from build123d import *

# Parameters (mm, degrees)
SALIENTE_EXTRUIR1_DEPTH = 5
CROQUIS3_W              = 12.5
CROQUIS3_H              = 5
SALIENTE_EXTRUIR2_DEPTH = 25
CROQUIS4_R              = 2.1
CORTAR_EXTRUIR3_DEPTH   = 12.5
CORTAR_EXTRUIR2_DEPTH   = 5.875


with BuildPart() as part:
    # Croquis2 → Saliente-Extruir1 (new body)
    with BuildSketch(Plane(origin=(0, 0, 0), x_dir=(1, 0, 0), z_dir=(0, 1, 0))):
        with BuildLine():
            Line((0, 0), (0, 12.5))
            Line((0, 12.5), (90, 35.865427318))
            add(Edge.make_bspline(
                [(0, 0), (0.394136999, 0.015797336), (1.194952966, 0.048834045), (2.992448828, 0.125211317), (4.579856068, 0.200911656), (6.612637351, 0.301249971), (8.392251736, 0.398752477), (10.315878033, 0.509903005), (12.159048858, 0.626310038), (14.511736704, 0.785189542), (17.305717547, 0.994336582), (20.114398042, 1.2314722), (22.909905137, 1.499776667), (25.707540494, 1.796493489), (29.430521004, 2.232380684), (34.457318955, 2.928516321), (39.917638309, 3.8880509), (45.326966885, 5.105084916), (49.769918493, 6.319079443), (53.346159155, 7.448006204), (56.870231766, 8.730995456), (60.329622828, 10.180098556), (63.710264837, 11.804910517), (66.997597592, 13.611491814), (70.17732587, 15.601579919), (72.854283587, 17.500893709), (75.067204078, 19.237089159), (76.854732505, 20.752585132), (78.250168573, 22.004629224), (79.619707974, 23.303249768), (80.962355597, 24.647453618), (82.277321506, 26.036087115), (83.403178931, 27.288894321), (84.345387571, 28.382707102), (85.115533062, 29.306902867), (85.722715368, 30.053623655), (86.321025458, 30.807421985), (86.910712224, 31.56828047), (87.491255325, 32.335040025), (88.06431213, 33.109755161), (88.629936117, 33.892108149), (89.099903233, 34.555740193), (89.55695597, 35.215829282), (89.829292977, 35.613909175), (89.943246974, 35.781569234), (90, 35.865427318)],
                knots=[0.074822974, 0.074822974, 0.074822974, 0.074822974, 0.074822974, 0.090398408, 0.105973841, 0.121549274, 0.137124708, 0.152700141, 0.168275574, 0.183851007, 0.199426441, 0.230577307, 0.261728173, 0.277303606, 0.29287904, 0.324029906, 0.386331636, 0.445924571, 0.477075434, 0.508226306, 0.539377159, 0.57052801, 0.601678868, 0.632829681, 0.663980451, 0.695131352, 0.726282194, 0.741857688, 0.757433182, 0.773008671, 0.788584161, 0.804576906, 0.820569651, 0.836562506, 0.844558934, 0.852555362, 0.860551891, 0.86854842, 0.87654495, 0.884541479, 0.89253801, 0.900534541, 0.908531072, 0.912529338, 0.916527603, 0.916527603, 0.916527603, 0.916527603, 0.916527603], degree=4))
        make_face()
    extrude(amount=SALIENTE_EXTRUIR1_DEPTH)

    # Croquis3 → Saliente-Extruir2 (add)
    with BuildSketch(Plane.ZY):
        with Locations((-6.25, 2.5)):
            Rectangle(CROQUIS3_W, CROQUIS3_H)
    extrude(amount=SALIENTE_EXTRUIR2_DEPTH)

    # Croquis4 → Cortar-Extruir3 (cut)
    with BuildSketch(Plane(origin=(0, 0, -12.5), x_dir=(-1, 0, 0), z_dir=(0, 0, -1))):
        with Locations((5, 2.5)):
            Circle(CROQUIS4_R)
    extrude(amount=-CORTAR_EXTRUIR3_DEPTH, mode=Mode.SUBTRACT)

    # Croquis5 → Cortar-Extruir2 (cut)
    with BuildSketch(Plane.XY):
        with BuildLine():
            Line((-16, 5), (-25, 5))
            Line((-25, 5), (-25, 0))
            Line((-25, 0), (-5, 0))
            ThreePointArc((-5, 0), (-7.5, 2.5), (-5, 5))
            Line((-5, 5), (-16, 5))
        make_face()
    extrude(amount=-CORTAR_EXTRUIR2_DEPTH, mode=Mode.SUBTRACT)


solid = part.part
Build history of the part. All positions in model axes, mm. A direction names the side the tool comes from. Round coordinates to 2 decimals unless told otherwise and drop trailing zeros. Order: outer loops, then holes, each group sorted by start corner. A loop starts at its lowest first (then second) coordinate and runs counter-clockwise, first axis right, second up. Notation, with made-up numbers: M 77.25,59 L 121.25,59 A19 cw 121.25,94 Z; hole C -7.75,-40 d6. An arc over 180 degrees is marked long. Use CSV: the item, a comma, the result in double quotes. Start each with the question number.
(1) Flat gauge pins, fed straight in: P1, Ø2, axis at y = 0.5, z = -26.5, coming from the +X side; P2, Ø10, axis at x = 47.5, z = -16.5, coming from the -Y side; P3, Ø2.5, axis at x = -5, y = 2.5, coming from the +Z side; P4, Ø2.5, axis at x = -18.5, y = 3.5, coming from the -Z side. Where does each tip first touch, or does it go through?
(2) Mould opens along X. For faces 4 (the face through (-25, 3, -9)), 5 (the face through (33, 0, -14)), 6 (the face through (-4.54, 0.45, -6.34)) say: +X half, -X half, draft (parallel to the pull), parting line (faces both ways), or undercut.
(3) Tool access for faces 1 (the face through (-2, 2, 0)), 2 (the face through (-7.5, 2.4, -2.9)), 3 (the face through (-12, 2, -12.5)): list every direction of +Z, -Z, +X, -X, +Y, -Y with a clear straight run to the whole face (end or side of a thin tool).
(4) Cut at A-A on x = -6. List the corners of the cut face in (y, z) (3 decimals), then the cut area to 3 significant figures.
(5) Drill centre lines: probe 1 along Y at (x, z) = (-5, -10); probe 2 along Z at (x, y) = (-2.5, 1.75); probe 3 along Z at (x, y) = (-18, 2.7) (3 decimals). Where is each one in solid material? Low to high.
Findings:
1,P1,"stops at x = 83.58"
1,P2,"stops at y = 0"
1,P3,"passes through"
1,P4,"stops at z = -12.5"
2,face 4,"-X half"
2,face 5,"draft"
2,face 6,"undercut"
3,face 1,"+Z, +X, -X, +Y, -Y"
3,face 2,"+Z, -X"
3,face 3,"-Z, -X, +Y, -Y"
4,outline,"M 0,-12.5 L 0.653,-12.5 L 0.653,0 L 0.209,0 L 0.209,-5.875 L 0,-5.875 Z; M 4.347,-12.5 L 5,-12.5 L 5,-5.875 L 4.791,-5.875 L 4.791,0 L 4.347,0 Z"
4,area,"13.9 mm^2"
5,probe 1,"y = 0 to 0.4, 4.6 to 5"
5,probe 2,"z = -12.5 to 0"
5,probe 3,"z = -12.5 to -5.875"
